The model under review builds one solid part; all positions refer to its coordinate system, in mm. Coordinates: 2 decimals unless noted, no trailing zeros. Loops run counter-clockwise (first coordinate to the right, second up) from the corner with the lowest first, then second, coordinate; pieces in that order, holes last. Notation, with made-up numbers: M 51.5,86.5 L 77.5,86.5 A17 ccw 77.5,101.5 Z; hole C 86,-14.5 d9. An arc over 180 degrees is marked long. Use one line per item in the form item = value.
```python
from build123d import *

# Parameters (mm, degrees)
SKETCH1_R          = 682.5
SKETCH1_R_2        = 652.5
BASE_FLANGE1_DEPTH = 2.5
SKETCH8_R          = 5
CUT_EXTRUDE1_DEPTH = 10


# Read off the part's stored shape, not the designer's step: Edge-Flange1
# Sheet-metal steps are written as plain solids
with BuildPart() as part:
    # Sketch1 → Base-Flange1 (new body)
    with BuildSketch(Plane(origin=(0, 0, 0), x_dir=(1, 0, 0), z_dir=(0, 1, 0))):
        with Locations(Location((0, 0, 0), (0, 0, 270))):
            Circle(SKETCH1_R)
        with Locations(Location((0, 0, 0), (0, 0, 270))):
            Circle(SKETCH1_R_2, mode=Mode.SUBTRACT)
    extrude(amount=-BASE_FLANGE1_DEPTH)

    # Edge-Flange1 outline → Edge-Flange1 (revolve, cut)
    with BuildSketch(Plane.XY):
        with BuildLine():
            Line((652.5, -2.5), (652.645898034, -2.5))
            ThreePointArc((652.645898034, -2.5), (653.908349934, -0.69375696), (656, 0))
            Line((656, 0), (652.5, 0))
            Line((652.5, 0), (652.5, -2.5))
        make_face()
    revolve(axis=Axis((0, 0, 0), (0, 1, 0)), mode=Mode.SUBTRACT)

    # Edge-Flange1 2 outline → Edge-Flange1 2 (revolve)
    with BuildSketch(Plane.XY):
        with BuildLine():
            Line((652.5, -3.5), (652.5, -33.5))
            Line((652.5, -33.5), (655, -33.5))
            Line((655, -33.5), (655, -3.5))
            ThreePointArc((655, -3.5), (655.292893219, -2.792893219), (656, -2.5))
            Line((656, -2.5), (652.645898034, -2.5))
            ThreePointArc((652.645898034, -2.5), (652.536666571, -2.994706462), (652.5, -3.5))
        make_face()
    revolve(axis=Axis((0, 0, 0), (0, 1, 0)))

    # Sketch8 → Cut-Extrude1 (cut)
    with BuildSketch(Plane(origin=(0, 0, 0), x_dir=(1, 0, 0), z_dir=(0, 1, 0))):
        with Locations(Location((172.761712606, 644.755489048, 0), (0, 0, 270))):
            Circle(SKETCH8_R)
        with Locations(Location((333.75, 578.071957026, 0), (0, 0, 270))):
            Circle(SKETCH8_R)
        with Locations(Location((0, 667.5, 0), (0, 0, 270))):
            Circle(SKETCH8_R)
        with Locations(Location((471.993776442, 471.993776442, 0), (0, 0, 270))):
            Circle(SKETCH8_R)
        with Locations(Location((578.071957026, 333.75, 0), (0, 0, 270))):
            Circle(SKETCH8_R)
        with Locations(Location((644.755489048, 172.761712606, 0), (0, 0, 270))):
            Circle(SKETCH8_R)
        with Locations(Location((667.5, 0, 0), (0, 0, 270))):
            Circle(SKETCH8_R)
        with Locations(Location((644.755489048, -172.761712606, 0), (0, 0, 270))):
            Circle(SKETCH8_R)
        with Locations(Location((578.071957026, -333.75, 0), (0, 0, 270))):
            Circle(SKETCH8_R)
        with Locations(Location((471.993776442, -471.993776442, 0), (0, 0, 270))):
            Circle(SKETCH8_R)
        with Locations(Location((333.75, -578.071957026, 0), (0, 0, 270))):
            Circle(SKETCH8_R)
        with Locations(Location((172.761712606, -644.755489048, 0), (0, 0, 270))):
            Circle(SKETCH8_R)
        with Locations(Location((0, -667.5, 0), (0, 0, 270))):
            Circle(SKETCH8_R)
        with Locations(Location((-172.761712606, -644.755489048, 0), (0, 0, 270))):
            Circle(SKETCH8_R)
        with Locations(Location((-333.75, -578.071957026, 0), (0, 0, 270))):
            Circle(SKETCH8_R)
        with Locations(Location((-471.993776442, -471.993776442, 0), (0, 0, 270))):
            Circle(SKETCH8_R)
        with Locations(Location((-578.071957026, -333.75, 0), (0, 0, 270))):
            Circle(SKETCH8_R)
        with Locations(Location((-644.755489048, -172.761712606, 0), (0, 0, 270))):
            Circle(SKETCH8_R)
        with Locations(Location((-667.5, 0, 0), (0, 0, 270))):
            Circle(SKETCH8_R)
        with Locations(Location((-644.755489048, 172.761712606, 0), (0, 0, 270))):
            Circle(SKETCH8_R)
        with Locations(Location((-578.071957026, 333.75, 0), (0, 0, 270))):
            Circle(SKETCH8_R)
        with Locations(Location((-471.993776442, 471.993776442, 0), (0, 0, 270))):
            Circle(SKETCH8_R)
        with Locations(Location((-333.75, 578.071957026, 0), (0, 0, 270))):
            Circle(SKETCH8_R)
        with Locations(Location((-172.761712606, 644.755489048, 0), (0, 0, 270))):
            Circle(SKETCH8_R)
    extrude(amount=-CUT_EXTRUDE1_DEPTH, mode=Mode.SUBTRACT)


solid = part.part
```
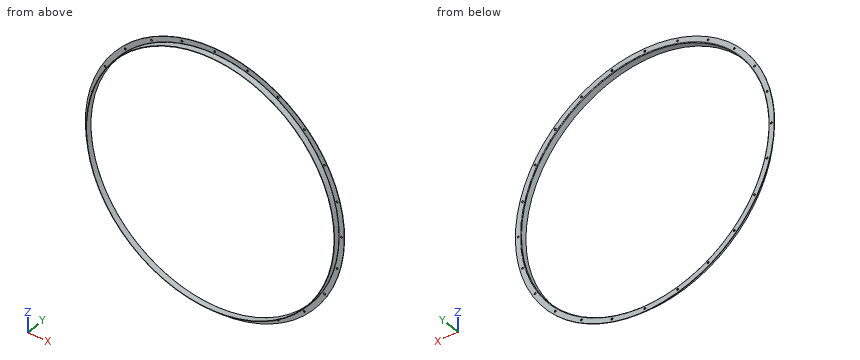
1. Wall thickness on line 1 along Z through (x, y) = (-333.75, -1.1); line 2 along X through (y, z) = (-1.9, -333.75); line 3 along Z through (x, y) = (333, -1): over which ranges is each line inside the solid? List them lowest first. Write a range as from..to.
Response values:
line_1 = -595.33..-583.07, -573.07..-561.79, 561.79..573.07, 583.07..595.33
line_2 = -595.33..-583.07, -573.07..-561.14, 561.14..573.07, 583.07..595.33
line_3 = -595.75..-583.02, -573.13..-562.35, 562.35..573.13, 583.02..595.75
2. Add section A-A (y = -11). State the section outline as (x, z) points.
Response values:
outline = C 0,0 d1310; hole C 0,0 d1305
3. Insertion check: P1, Ø9, axis at x = 0, z = -667.5, coming from the +Y side; P2, Ø11.5, axis at x = 471.99, z = 471.99, coming from the -Y side; P3, Ø8, axis at y = -21.5, z = 330.5, coming from the +X side; P4, Ø2, axis at x = 156, y = -7, coming from the -Z side. Each pin has a flat end and moves straight along its axis. Give the tip position at first contact, or say it passes through.
Response values:
P1 = through
P2 = -2.5
P3 = 567.82
P4 = -636.4
